```python
from build123d import *

# Parameters (mm, degrees)
SKETCH1_R           = 1.6
BOSS_EXTRUDE1_DEPTH = 5


with BuildPart() as part:
    # Sketch1 → Boss-Extrude1 (new body)
    with BuildSketch(Plane(origin=(0, 0, 0), x_dir=(1, 0, 0), z_dir=(0, 1, 0))):
        Polygon((-19, 4), (19, 4), (19, -12), (-19, -12), (-19, -4), align=None)
        with Locations((-7, 1)):
            Circle(SKETCH1_R, mode=Mode.SUBTRACT)
        with Locations((7, 1)):
            Circle(SKETCH1_R, mode=Mode.SUBTRACT)
        with Locations((15.1, 0)):
            Circle(SKETCH1_R, mode=Mode.SUBTRACT)
        with Locations((-15.1, 0)):
            Circle(SKETCH1_R, mode=Mode.SUBTRACT)
        with Locations((-15.1, -8)):
            Circle(SKETCH1_R, mode=Mode.SUBTRACT)
        with Locations((15.1, -8)):
            Circle(SKETCH1_R, mode=Mode.SUBTRACT)
        with Locations((7, -9)):
            Circle(SKETCH1_R, mode=Mode.SUBTRACT)
        with Locations((-7, -9)):
            Circle(SKETCH1_R, mode=Mode.SUBTRACT)
    extrude(amount=BOSS_EXTRUDE1_DEPTH)


solid = part.part
```
Can you work these out from the model? Positions are in its coordinate system, mm. Give positions to 0.01 mm unless a question says otherwise; leave off trailing zeros. Loops run counter-clockwise (first coordinate to the right, second up) from the corner with the lowest first, then second, coordinate; pieces in that order, holes last. Notation, with made-up numbers: M 46,-19 L 88,-19 A23 ccw 88,9 Z; hole C 28,-4.75 d5. An arc over 180 degrees is marked long. Use one line per item in the form item = value. Start each with the question number.
(1) I'm going to push flat-ended pins straight in: P1, Ø3, axis at x = -15.1, z = 8, coming from the +Y side; P2, Ø1, axis at x = -4.5, z = 9, coming from the -Y side. Where does each tip first touch, or does it pass through?
(2) I want a section at A-A, the plane x = 15.1. Write out the boundary of the cut face in (y, z).
(3) Please list where these lines run through material, in increasing order: line 1 (Z direction, x = 7, y = 2.05); line 2 (X direction, y = 2.35, z = 8); line 3 (X direction, y = 3.9, z = 0.75).
(4) Thinking about a two-plate mould opening in X: for faces 1 (the flat face through (0, 0, 4)), 2 (the flat face through (-19, 2, 4)), 3 (the cylindrical face through (5.4, 2.46, -1.07)), 4 (the cylindrical face through (-13.574, 2.465, -0.481)), which applies, released by +X, released by -X, zero draft, split by the parting line, or undercut?
(5) I want a section at B-B, the plane y = 3.7. State how many separate pieces and enclosed holes the cut face has, and give its area (3 significant figures).
(6) I want a section at C-C, the plane z = 0. Write out the boundary of the cut face in (x, y), and give its area (3 significant figures).
(7) I want a section at D-D, the plane z = 6.75. Write out the boundary of the cut face in (x, y), and give its area (3 significant figures).
Worked out:
q1.P1 = through
q1.P2 = 0
q2.outline = M 0,-4 L 5,-4 L 5,-1.6 L 0,-1.6 Z; M 0,1.6 L 5,1.6 L 5,6.4 L 0,6.4 Z; M 0,9.6 L 5,9.6 L 5,12 L 0,12 Z
q3.line_1 = -4 to -2.6, 0.6 to 7.4, 10.6 to 12
q3.line_2 = -19 to -16.7, -13.5 to -8.25, -5.75 to 5.75, 8.25 to 13.5, 16.7 to 19
q3.line_3 = -19 to -16.51, -13.69 to 13.69, 16.51 to 19
q4.face_1 = zero draft
q4.face_2 = released by -X
q4.face_3 = undercut
q4.face_4 = undercut
q5.separate_pieces = 1
q5.enclosed_holes = 8
q5.area = 544 mm²
q6.outline = M -19,0 L -16.7,0 L -16.7,5 L -19,5 Z; M -13.5,0 L -8.25,0 L -8.25,5 L -13.5,5 Z; M -5.75,0 L 5.75,0 L 5.75,5 L -5.75,5 Z; M 8.25,0 L 13.5,0 L 13.5,5 L 8.25,5 Z; M 16.7,0 L 19,0 L 19,5 L 16.7,5 Z
q6.area = 133 mm²
q7.outline = M -19,0 L -16.1,0 L -16.1,5 L -19,5 Z; M -14.1,0 L 14.1,0 L 14.1,5 L -14.1,5 Z; M 16.1,0 L 19,0 L 19,5 L 16.1,5 Z
q7.area = 170 mm²
